Part model, mm, in its own coordinate system. Face numbers are marked on the shaded views. A direction names the side the tool comes from. Give positions to 0.01 mm unless a question says otherwise; leave off trailing zeros. Order: outer loops, then holes, each group sorted by start corner. A loop starts at its lowest first (then second) coordinate and runs counter-clockwise, first axis right, second up. Notation, with made-up numbers: (-30, -17) - (-15, -17) arc R7 cw to (-15, -7) - close; hole circle Ø6 at (56, 40). An arc over 180 degrees is marked (long way). One line per item, written item: value.
```python
from build123d import *

# Parameters (mm, degrees)
SKETCH1_W           = 16
SKETCH1_H           = 56
SKETCH1_W_2         = 10
SKETCH1_H_2         = 50
EXTRUDE_THIN1_DEPTH = 80
SKETCH2_R           = 13
SKETCH2_R_2         = 2
CUT_EXTRUDE1_DEPTH  = 17


with BuildPart() as part:
    # Sketch1 → Extrude-Thin1 (new body)
    with BuildSketch(Plane(origin=(0, 0, 0), x_dir=(1, 0, 0), z_dir=(0, 1, 0))):
        Rectangle(SKETCH1_W, SKETCH1_H)
        Rectangle(SKETCH1_W_2, SKETCH1_H_2, mode=Mode.SUBTRACT)
    extrude(amount=EXTRUDE_THIN1_DEPTH)

    # Sketch2 → Cut-Extrude1 (cut, through all)
    with BuildSketch(Plane.ZY.offset(8)):
        with Locations((0, 50)):
            Circle(SKETCH2_R)
        with Locations((-24.79735893, 4.015533462)):
            Circle(SKETCH2_R_2)
        with Locations((-14.79735893, 4.015533462)):
            Circle(SKETCH2_R_2)
        with Locations((-4.79735893, 4.015533462)):
            Circle(SKETCH2_R_2)
        with Locations((5.20264107, 4.015533462)):
            Circle(SKETCH2_R_2)
        with Locations((15.20264107, 4.015533462)):
            Circle(SKETCH2_R_2)
        with Locations((25.20264107, 4.015533462)):
            Circle(SKETCH2_R_2)
        with Locations((-14.79735893, 14.015533462)):
            Circle(SKETCH2_R_2)
        with Locations((-4.79735893, 14.015533462)):
            Circle(SKETCH2_R_2)
        with Locations((5.20264107, 14.015533462)):
            Circle(SKETCH2_R_2)
        with Locations((15.20264107, 14.015533462)):
            Circle(SKETCH2_R_2)
        with Locations((25.20264107, 14.015533462)):
            Circle(SKETCH2_R_2)
        with Locations((-24.79735893, 14.015533462)):
            Circle(SKETCH2_R_2)
    extrude(amount=-CUT_EXTRUDE1_DEPTH, mode=Mode.SUBTRACT)


solid = part.part
```
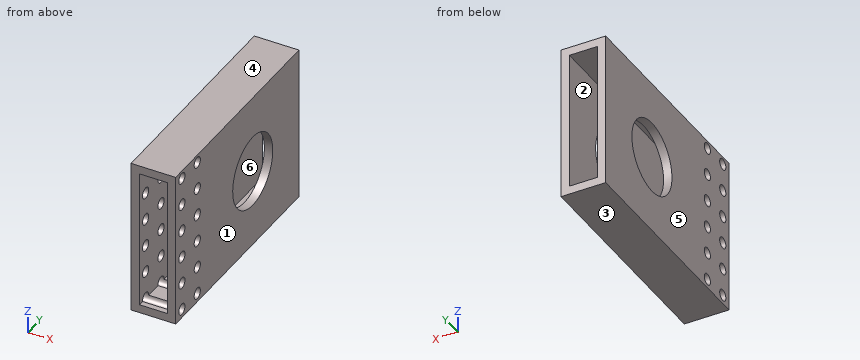
1) Mould opens along Z. For the marked faces 1, 2, 3 and 4 say: released by +Z, released by -Z, zero draft, split by the parting line, or undercut.
Outcome:
face 1: zero draft
face 2: undercut
face 3: released by -Z
face 4: released by +Z
2) Cut at C-C, the plane y = 50. Give the cut face in (x, z), then the cut area to 3 significant figures.
Outcome:
outline: (-8, -28) - (8, -28) - (8, -13) - (5, -13) - (5, -25) - (-5, -25) - (-5, -13) - (-8, -13) - close; (-8, 13) - (-5, 13) - (-5, 25) - (5, 25) - (5, 13) - (8, 13) - (8, 28) - (-8, 28) - close
area: 240 mm^2
3) Which spindle directions (+Z, -Z, +X, -X, +Y, -Y) get a long thin tool onto all of the face, cutting with end or side? Do the marked faces 5 and 6. Say none if no direction does.
Outcome:
face 5: +Z, -Z, -X, +Y, -Y
face 6: +Y, -Y
4) Cut at B-B, the plane z = 0. Give the cut face in (x, y), then the cut area to 3 significant figures.
Outcome:
outline: (-8, 0) - (-5, 0) - (-5, 37) - (-8, 37) - close; (-8, 63) - (-5, 63) - (-5, 80) - (-8, 80) - close; (5, 0) - (8, 0) - (8, 37) - (5, 37) - close; (5, 63) - (8, 63) - (8, 80) - (5, 80) - close
area: 324 mm^2
5) Cut at D-D, the plane y = 35. Give the cut face in (x, z), then the cut area to 3 significant figures.
Outcome:
outline: (-8, -28) - (8, -28) - (8, 28) - (-8, 28) - close; hole (-5, -25) - (5, -25) - (5, 25) - (-5, 25) - close
area: 396 mm^2
6) Cut at A-A, the plane x = 3.25. Give the cut face in (y, z), then the cut area to 3 significant figures.
Outcome:
outline: (0, -28) - (80, -28) - (80, -25) - (16.01, -25) arc R2 cw to (12.03, -25) - (6.01, -25) arc R2 cw to (2.03, -25) - (0, -25) - close; (0, 25) - (2.03, 25) arc R2 cw (long way) to (6.01, 25) - (12.03, 25) arc R2 cw (long way) to (16.01, 25) - (80, 25) - (80, 28) - (0, 28) - close
area: 455 mm^2
7) Drill centre lines: line 1 along X through (y, z) = (9.5, 11); line 2 along Z through (x, y) = (0, 68); line 3 along Y through (x, z) = (-3, 26). Where is each one in solid material? Low to high. Write a range as from..to.
Outcome:
line 1: x = -8..-5, 5..8
line 2: z = -28..-25, 25..28
line 3: y = 0..2.18, 5.85..12.18, 15.85..80
8) Pin check, flat tip, straight feed: pin 1 (3 mm diameter, centred on x = 0, z = 22, fed in from +Y). Stop position of the tip, or through.
Outcome:
pin 1: passes through
